Input: dimensioned drawing with shaded views. Units: mm. Origin: part minimum x, y, z. A direction names the side the tool comes from. Round coordinates to 2 decimals unless told otherwise and drop trailing zeros. Order: outer loops, then holes, each group sorted by start corner. A loop starts at its lowest first (then second) coordinate and runs counter-clockwise, first axis right, second up.
Item 1: Cut plane D-D on y = 17. Output: boundary loops of the cut face in (x, z), then the cut area to 3 significant figures.
Item 2: First-contact query: pin 1 (1.5 mm diameter, centred on x = 24, y = 34.5, fed in from -Z); pin 2 (5 mm diameter, centred on x = 7, z = 11.5, fed in from +Y); pin 3 (4 mm diameter, centred on x = 23, y = 48.5, fed in from +Z). Flat tips, straight axial feed; report the tip coordinate or a pass-through.
Item 3: Line query: L1, parallel to X at y = 28, z = 19.5; L2, parallel to Y at x = 16, z = 38.5; L3, parallel to Y at x = 35.5, z = 31. Output: solid intervals per line, ascending.
Item 4: Cut plane A-A on z = 41.91. Output: boundary loops of the cut face in (x, y), then the cut area to 3 significant figures.
Item 5: Mould query, pull axis X, two halves, no side actions, for the marked faces 1, 2 and 3. Classes: released by +X, released by -X, zero draft, split by the parting line, or undercut.
Item 6: Cut plane B-B on z = 62.5. Output: boundary loops of the cut face in (x, y), then the cut area to 3 significant figures.
Item 7: Reachability of the marked faces 4 and 5 from +Z, -Z, +X, -X, +Y, -Y: full face, straight path, thin tool, end or side. Return the list, or none.
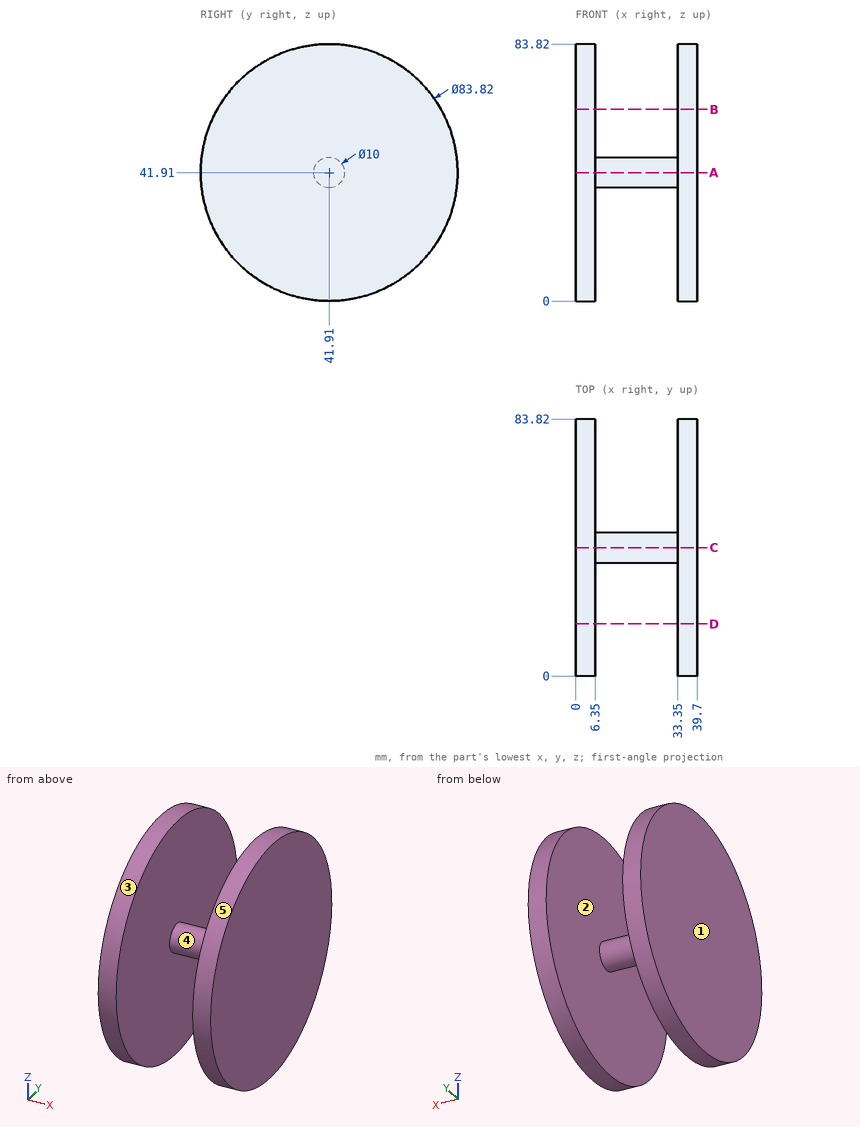
From the geometry:
1. outline: (0, 8.21) - (6.35, 8.21) - (6.35, 75.61) - (0, 75.61) - close; (33.35, 8.21) - (39.7, 8.21) - (39.7, 75.61) - (33.35, 75.61) - close
1. area: 856 mm2
2. pin 1: passes through
2. pin 2: stops at y = 73.1
2. pin 3: stops at z = 43.89
3. L1: x = 0 to 6.35, 33.35 to 39.7
3. L2: y = 38.25 to 45.57
3. L3: y = 1.44 to 82.38
4. outline: (0, 0) - (6.35, 0) - (6.35, 36.91) - (33.35, 36.91) - (33.35, 0) - (39.7, 0) - (39.7, 83.82) - (33.35, 83.82) - (33.35, 46.91) - (6.35, 46.91) - (6.35, 83.82) - (0, 83.82) - close
4. area: 1,330 mm2
5. face 1: released by -X
5. face 2: undercut
5. face 3: zero draft
6. outline: (0, 5.41) - (6.35, 5.41) - (6.35, 78.41) - (0, 78.41) - close; (33.35, 5.41) - (39.7, 5.41) - (39.7, 78.41) - (33.35, 78.41) - close
6. area: 927 mm2
7. face 4: none
7. face 5: +X, -X
